Verification items for this drawing (mm, ordinates from the low corner). A direction names the side the tool comes from. Round coordinates to 2 decimals unless told otherwise and drop trailing zeros. Order: outer loops, then holes, each group sorted by start corner. A loop starts at its lowest first (then second) coordinate and runs counter-clockwise, first axis right, second up. Notation, with made-up numbers: (46, 86.25) - (54, 86.25) arc R19 ccw to (54, 122.25) - close; hole circle Ø4 at (13, 84). An arc over 180 degrees is marked (long way). Use a Markdown table: item, result. Add a question column.
(1) Section check B-B on y = 81. Record the boundary of the cut face in (x, z), then the cut area to 3 significant figures.
(2) Access from +Z, -Z, +X, -X, +Y, -Y to the whole of each face (thin tool, end or side, straight path). Record for the marked faces 4 and 5.
(3) Section check C-C on z = 52.5. Record the boundary of the cut face in (x, y).
(4) Gauge pin test, flat ends, axial feed: P1, Ø3, axis at x = 75, z = 130, coming from the -Y side; P2, Ø3, axis at x = 80.5, z = 124.5, coming from the -Y side; P3, Ø9.5, axis at x = 4.5, z = 80, coming from the -Y side; P4, Ø7, axis at x = 40, y = 65, coming from the +Z side. Record the tip position at first contact, or that the pin passes through.
(5) Mould release check, pull along Z, two halves, no side actions. Record for the marked faces 1, 2 and 3: released by +Z, released by -Z, zero draft, split by the parting line, or undercut.
(6) Section check A-A on y = 65. Record the boundary of the cut face in (x, z), then the cut area to 3 significant figures.
(7) Thickness scan on line 1 along X through (y, z) = (107, 75); line 2 along Y through (x, z) = (40, 140); line 3 along X through (y, z) = (79, 127). Record the ranges inside material, lowest first. Write a range as [from, to].
(8) Section check D-D on y = 103.5. Record the boundary of the cut face in (x, z), then the cut area to 3 significant figures.
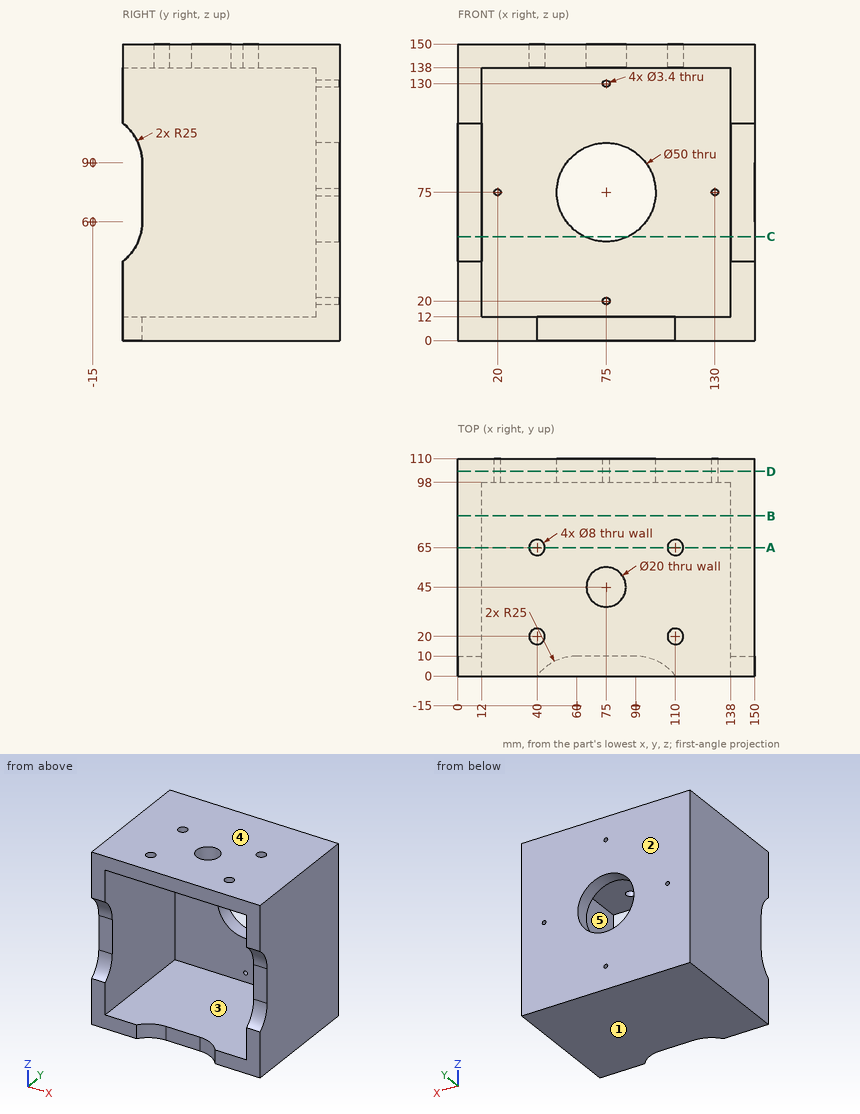
Check sheet entries:
| question | item | result |
|---|---|---|
| 1 | outline | (0, 0) - (150, 0) - (150, 150) - (0, 150) - close; hole (12, 12) - (138, 12) - (138, 138) - (12, 138) - close |
| 1 | area | 6,620 mm2 |
| 2 | face 4 | +Z, +X, -X, +Y, -Y |
| 2 | face 5 | -Y |
| 3 | outline | (0, 8.85) - (12, 8.85) - (12, 98) - (64.1, 98) - (64.1, 110) - (0, 110) - close; (85.9, 98) - (138, 98) - (138, 8.85) - (150, 8.85) - (150, 110) - (85.9, 110) - close |
| 4 | P1 | passes through |
| 4 | P2 | stops at y = 98 |
| 4 | P3 | stops at y = 10 |
| 4 | P4 | stops at z = 12 |
| 5 | face 1 | released by -Z |
| 5 | face 2 | zero draft |
| 5 | face 3 | undercut |
| 6 | outline | (0, 0) - (150, 0) - (150, 150) - (114, 150) - (114, 138) - (138, 138) - (138, 12) - (12, 12) - (12, 138) - (36, 138) - (36, 150) - (0, 150) - close; (44, 138) - (106, 138) - (106, 150) - (44, 150) - close |
| 6 | area | 6,430 mm2 |
| 7 | line 1 | x = [0, 18.3], [21.7, 50], [100, 128.3], [131.7, 150] |
| 7 | line 2 | y = [0, 16], [24, 61], [69, 110] |
| 7 | line 3 | x = [0, 12], [138, 150] |
| 8 | outline | (0, 0) - (150, 0) - (150, 150) - (0, 150) - close; hole circle Ø3.4 at (20, 75); hole circle Ø50 at (75, 75); hole circle Ø3.4 at (75, 20); hole circle Ø3.4 at (75, 130); hole circle Ø3.4 at (130, 75) |
| 8 | area | 20,500 mm2 |
